Input: part model. Units: mm. Frame: model coordinates. Face numbers are marked on the shaded views. A direction names the side the tool comes from. Give positions to 0.01 mm unless a question says otherwise; leave off trailing zeros. Loops run counter-clockwise (first coordinate to the right, second up) from the corner with the lowest first, then second, coordinate; pieces in that order, holes last.
from build123d import *

# Parameters (mm, degrees)
PAD016_DEPTH = 50
PAD017_DEPTH = 2
PAD018_DEPTH = 10
PAD019_DEPTH = 3
FILLET_R     = 1
FILLET001_R  = 3
FILLET002_R  = 2


with BuildPart() as part:
    # Sketch024 → Pad016 (new body)
    with BuildSketch(Plane.XY):
        with BuildLine():
            Line((0, 0), (150, 0))
            ThreePointArc((150, 0), (175.963449, 27.378164), (147.247546, 51.853897))
            ThreePointArc((147.247546, 51.853897), (129.103193, 80.569725), (95.135939, 80.364888))
            ThreePointArc((95.135939, 80.364888), (46.395903, 117.272917), (5.84043, 71.523082))
            ThreePointArc((5.84043, 71.523082), (-35.880572, 38.929935), (0, 0))
        make_face()
        with BuildLine():
            ThreePointArc((92.566341, 74.797944), (47.150665, 114.129661), (9.33601, 67.443265))
            ThreePointArc((9.33601, 67.443265), (-32.459044, 40.717039), (0, 3.2))
            Line((0, 3.2), (150, 3.2))
            ThreePointArc((150, 3.2), (172.60162, 29.001128), (144.049968, 48.009932))
            ThreePointArc((144.049968, 48.009932), (126.982256, 78.074612), (92.566341, 74.797944))
        make_face(mode=Mode.SUBTRACT)
    extrude(amount=PAD016_DEPTH)

    # Sketch025 (on Face12 of Pad016) → Pad017 (join)
    with BuildSketch(Plane.XY.offset(50)):
        with BuildLine():
            Line((0, 0), (150, 0))
            ThreePointArc((150, 0), (175.963449, 27.378164), (147.247546, 51.853897))
            ThreePointArc((147.247546, 51.853897), (129.103193, 80.569725), (95.135939, 80.364888))
            ThreePointArc((95.135939, 80.364888), (46.395903, 117.272917), (5.84043, 71.523082))
            ThreePointArc((5.84043, 71.523082), (-35.880572, 38.929935), (0, 0))
        make_face()
        with BuildLine():
            ThreePointArc((87.815114, 71.442447), (48.520032, 109.41973), (14.263984, 66.841559))
            Line((8.892558, 62.550375), (14.263984, 66.841559))
            ThreePointArc((8.892558, 62.550375), (-27.635218, 40.504969), (0, 8))
            Line((0, 8), (150, 8))
            ThreePointArc((150, 8), (167.729763, 29.107329), (143.878644, 42.927168))
            Line((139.179868, 47.277594), (143.878644, 42.927168))
            ThreePointArc((139.179868, 47.277594), (123.936648, 74.230459), (93.393809, 69.136577))
            Line((87.815114, 71.442447), (93.393809, 69.136577))
        make_face(mode=Mode.SUBTRACT)
    extrude(amount=PAD017_DEPTH)

    # Sketch026 (on Face15 of Pad017) → Pad018 (join)
    with BuildSketch(Plane.XY.offset(52)):
        with BuildLine():
            Line((0, 0), (150, 0))
            ThreePointArc((150, 0), (175.963449, 27.378164), (147.247546, 51.853897))
            ThreePointArc((147.247546, 51.853897), (129.103193, 80.569725), (95.135939, 80.364888))
            ThreePointArc((95.135939, 80.364888), (46.395903, 117.272917), (5.84043, 71.523082))
            ThreePointArc((5.84043, 71.523082), (-35.880572, 38.929935), (0, 0))
        make_face()
        with BuildLine():
            ThreePointArc((92.566341, 74.797944), (47.150665, 114.129661), (9.33601, 67.443265))
            ThreePointArc((9.33601, 67.443265), (-32.459044, 40.717039), (0, 3.2))
            Line((0, 3.2), (150, 3.2))
            ThreePointArc((150, 3.2), (172.60162, 29.001128), (144.049968, 48.009932))
            ThreePointArc((144.049968, 48.009932), (126.982256, 78.074612), (92.566341, 74.797944))
        make_face(mode=Mode.SUBTRACT)
    extrude(amount=PAD018_DEPTH)

    # Sketch027 (on Face21 of Pad018) → Pad019 (join)
    with BuildSketch(Plane.XY.offset(62)):
        with BuildLine():
            Line((0, 0), (150, 0))
            ThreePointArc((150, 0), (175.963449, 27.378164), (147.247546, 51.853897))
            ThreePointArc((147.247546, 51.853897), (129.103193, 80.569725), (95.135939, 80.364888))
            ThreePointArc((95.135939, 80.364888), (46.395903, 117.272917), (5.84043, 71.523082))
            ThreePointArc((5.84043, 71.523082), (-35.880572, 38.929935), (0, 0))
        make_face()
        with BuildLine():
            ThreePointArc((84.015068, 61.367554), (47.028893, 107.28489), (20.829728, 54.464603))
            Line((19.480393, 53.219591), (20.829728, 54.464603))
            ThreePointArc((19.480393, 53.219591), (-23.703474, 46.683881), (0, 10))
            Line((0, 10), (150, 10))
            ThreePointArc((150, 10), (164.62434, 32.490661), (138.134796, 36.733915))
            Line((134.91887, 39.207776), (138.134796, 36.733915))
            ThreePointArc((134.91887, 39.207776), (122.444141, 72.716079), (89.228181, 59.48259))
            Line((84.015068, 61.367554), (89.228181, 59.48259))
        make_face(mode=Mode.SUBTRACT)
    extrude(amount=PAD019_DEPTH)

    # Fillet
    fillet_edges = [part.edges().sort_by_distance(p)[0] for p in [
        (20.829728, 54.464603, 63.5),
        (19.480393, 53.219591, 63.5),
    ]]
    fillet(fillet_edges, radius=FILLET_R)

    # Fillet001
    fillet001_edges = [part.edges().sort_by_distance(p)[0] for p in [
        (89.228181, 59.48259, 63.5),
        (84.015068, 61.367554, 63.5),
    ]]
    fillet(fillet001_edges, radius=FILLET001_R)

    # Fillet002
    fillet002_edges = [part.edges().sort_by_distance(p)[0] for p in [
        (138.134796, 36.733915, 63.5),
        (134.91887, 39.207776, 63.5),
    ]]
    fillet(fillet002_edges, radius=FILLET002_R)


with BuildPart() as part_1:
    # Body004 placement: moved
    add(part.part.moved(Location((-11.904526, 86.281793, 0))))


solid = part_1.part
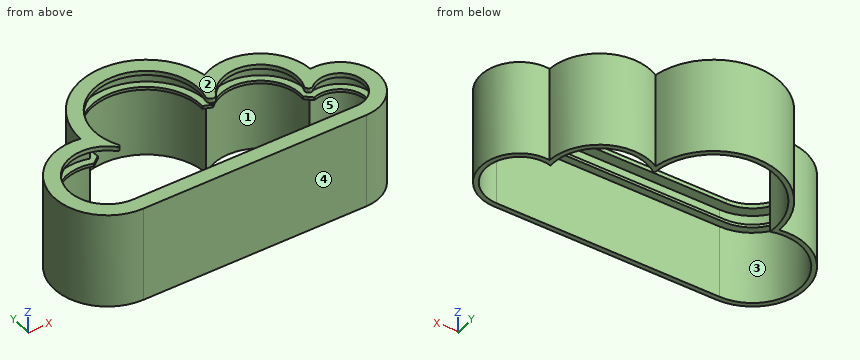
(1) Reachability of the marked faces 1 and 2 from +Z, -Z, +X, -X, +Y, -Y: full face, straight path, thin tool, end or side. Return the list, or none.
Values follow:
face 1: -Z
face 2: +Z, +X, -X, +Y, -Y
(2) Ray query, probe 1 along Z at (x, y) = (39, 93); probe 2 along Y at (x, z) = (122, 39); probe 3 along Y at (x, z) = (139.5, 7.5). Return the intervals inside material, ascending.
Values follow:
probe 1: z = 50 to 52, 62 to 65
probe 2: y = 86.28 to 89.48, 159.48 to 163.69
probe 3: y = 86.32 to 89.53, 135.04 to 138.24
(3) Mould query, pull axis X, two halves, no side actions, for the marked faces 3, 4 and 5. Classes: +X half, -X half, draft (parallel to the pull), parting line (faces both ways), or undercut.
Values follow:
face 3: undercut
face 4: draft
face 5: undercut
(4) Cut plane C-C (z = 13). Return the cut outline in (x, y), and give its area (3 significant figures).
Values follow:
outline: (-11.9, 86.28) - (138.1, 86.28) arc R26 ccw (long way) to (135.34, 138.14) arc R35 ccw to (83.23, 166.65) arc R45 ccw to (-6.06, 157.8) arc R36 ccw (long way) to start; hole (-11.9, 89.48) - (138.1, 89.48) arc R22.8 ccw (long way) to (132.15, 134.29) arc R31.8 ccw to (80.66, 161.08) arc R41.8 ccw (long way) to (-2.57, 153.73) arc R32.8 ccw (long way) to start
area: 1,770 mm2
(5) Cut plane A-A (y = 112). Return the cut outline in (x, z), and give its area (3 significant figures).
Values follow:
outline: (-46.41, 0) - (-43.05, 0) - (-43.05, 50) - (-37.95, 50) - (-37.95, 52) - (-43.05, 52) - (-43.05, 62) - (-35.79, 62) - (-35.79, 65) - (-46.41, 65) - close; (154.09, 62) - (160.89, 62) - (160.89, 52) - (156.09, 52) - (156.09, 50) - (160.89, 50) - (160.89, 0) - (164.09, 0) - (164.09, 65) - (154.09, 65) - close
area: 488 mm2
(6) Cut plane B-B (x = 21). Return the cut outline in (y, z), and give its area (3 significant figures).
Values follow:
outline: (86.28, 0) - (89.48, 0) - (89.48, 50) - (94.28, 50) - (94.28, 52) - (89.48, 52) - (89.48, 62) - (96.28, 62) - (96.28, 65) - (86.28, 65) - close; (188.83, 62) - (196.54, 62) - (196.54, 52) - (191.14, 52) - (191.14, 50) - (196.54, 50) - (196.54, 0) - (200.05, 0) - (200.05, 65) - (188.83, 65) - close
area: 500 mm2
(7) Pin query (flat end, axial travel): pin 1 Ø2 at (x, z) = (-14, 15) entering from +Y; pin 2 Ø1 at (y, z) = (146.5, 38.5) entering from -X; pin 3 Ø3.5 at (x, z) = (32, 63) entering from +Y. Return the tip coordinate at first contact, or that it passes through.
Values follow:
pin 1: stops at y = 158.27
pin 2: stops at x = -38.99
pin 3: stops at y = 203.48
